Input: part model. Units: mm. Frame: model coordinates. A direction names the side the tool comes from. Coordinates: 2 decimals unless noted, no trailing zeros. Order: outer loops, then holes, each group sorted by start corner. A loop starts at its lowest first (then second) coordinate and runs counter-clockwise, first axis right, second up. Notation, with made-up numbers: (25, 11) - (42, 11) arc R33 cw to (42, 48) - close; hole circle Ø8 at (9.5, 43.5). An arc over 180 degrees is marked (long way). One line per question, with ' | ' between items.
from build123d import *

# Parameters (mm, degrees)
SKETCH171_R          = 1.55
POCKET093_DEPTH      = 10.0010001
POCKET093_DEPTH_BACK = 10.0010001
SKETCH183_R          = 1.6
POCKET099_DEPTH      = 5


with BuildPart() as part:
    # Sketch169 → AdditiveLoft006 section 0
    with BuildSketch(Plane.XY):
        Polygon((-15, -10), (15, -10), (15, -6), (-11, -6), (-11, 10), (-15, 10), align=None)
    # Sketch170 → AdditiveLoft006 section 1
    with BuildSketch(Plane(origin=(-12, 0, 20), x_dir=(1, 0, 0), z_dir=(0, 0, 1))):
        Polygon((-15, -10), (15, -10), (15, -6), (-11, -6), (-11, 10), (-15, 10), align=None)
    loft()

    # Sketch171 → Pocket093 (cut, two sides)
    with BuildSketch(Plane.XZ) as pocket093_sk:
        with Locations((-4, 10)):
            Circle(SKETCH171_R)
    extrude(amount=-POCKET093_DEPTH, mode=Mode.SUBTRACT)
    extrude(pocket093_sk.sketch, amount=POCKET093_DEPTH_BACK, mode=Mode.SUBTRACT)

    # Sketch183 (on Face5 of Pocket093) → Pocket099 (cut)
    with BuildSketch(Plane(origin=(-8.0882352941, 0, -4.8529411765), x_dir=(0, 1, 0), z_dir=(0.8574929257, 0, 0.5144957554))):
        with Locations((0, 17.3213533097)):
            Circle(SKETCH183_R)
    extrude(amount=-POCKET099_DEPTH, mode=Mode.SUBTRACT)


solid = part.part
Item 1: Contact query for flat-ended pins moving along their axis: P1, Ø5, axis at x = -10, y = -2.5, coming from the +Z side; P2, Ø5, axis at y = -5, z = 12.5, coming from the +X side; P3, Ø4, axis at x = -4, z = 10, coming from the +Y side. Output: stop coordinate, or through.
Data:
P1: z = 2.5 | P2: x = 8.87 | P3: y = -6
Item 2: Ray query, line 1 (Z direction, x = -4, y = -7.75); line 2 (Y direction, x = 3.5, z = 4); line 3 (X direction, y = -6.8, z = 10). Return the intervals inside material, ascending.
Data:
line 1: 0 to 8.45, 11.55 to 20 | line 2: -10 to -6 | line 3: -21 to -5.55, -2.45 to 9
Item 3: Section B-B on y = 5.25. Return the cut outline in (x, z).
Data:
outline: (-27, 20) - (-15, 0) - (-11, 0) - (-23, 20) - close
Item 4: Section A-A on y = -8.25. Return the cut outline in (x, z), and give its area (3 significant figures).
Data:
outline: (-27, 20) - (-15, 0) - (15, 0) - (3, 20) - close; hole circle Ø3.1 at (-4, 10) | area: 592 mm^2
Item 5: Draft query along Y for faces 1 (the face through (-17.65, -0.35, 7.79)), 2 (the face through (-5.23, -7.97, 9.06)). Return one class per face: released by +Y, released by -Y, zero draft, split by the parting line, or undercut.
Data:
face 1: undercut | face 2: zero draft
Item 6: Access query for faces 3 (the face through (-17, 2, 10)), 4 (the face through (-15, -7, 20)). Directions: +Z, -Z, +X, -X, +Y, -Y. A direction counts if a zero-diameter tool reaches every point of the face in a straight line with its end or side. Return the directions, or none.
Data:
face 3: +Z, +X, +Y | face 4: +Z, +X, -X, +Y, -Y
